Design review of the part shown in the three views and the two pictorial views. Dimensions are in mm from the part's minimum x, y and z. Round coordinates to 2 decimals unless told otherwise and drop trailing zeros. Loops run counter-clockwise (first coordinate to the right, second up) from the corner with the lowest first, then second, coordinate; pieces in that order, holes last.
1) Insertion check: pin 1 (8 mm diameter, centred on x = 7, y = 21, fed in from -Z); pin 2 (0.5 mm diameter, centred on y = 7, z = 0.5, fed in from -X). Each pin has a flat end and moves straight along its axis. Give the tip position at first contact, or say it passes through.
2) Take a section at A-A (z = 0.3). State the section outline as (x, y) points, then the cut area to 3 significant figures.
3) Take a section at B-B (y = 12.75). State the section outline as (x, z) points, then the cut area to 3 significant figures.
4) Wall thickness on L1, parallel to X at y = 2.75, z = 0.6; L2, parallel to Y at x = 2.5, z = 0.25: over which ranges is each line inside the solid? List them lowest first.
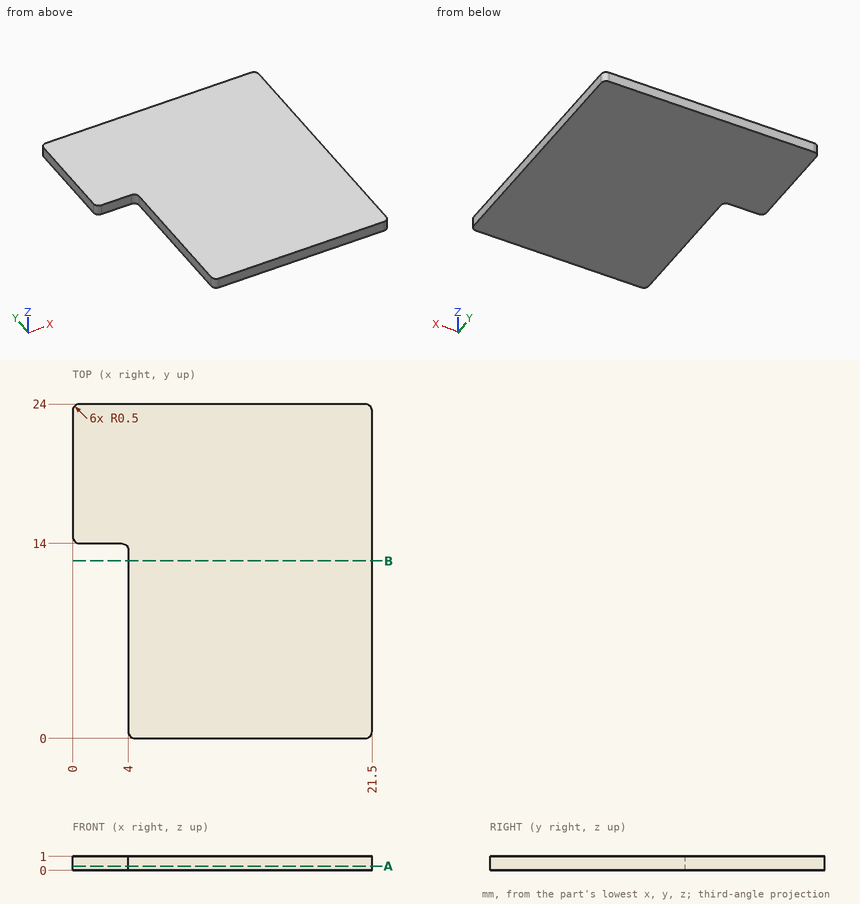
Response:
1. pin 1: stops at z = 0
1. pin 2: stops at x = 4
2. outline: (0, 14.5) arc R0.5 ccw to (0.5, 14) - (3.5, 14) arc R0.5 cw to (4, 13.5) - (4, 0.5) arc R0.5 ccw to (4.5, 0) - (21, 0) arc R0.5 ccw to (21.5, 0.5) - (21.5, 23.5) arc R0.5 ccw to (21, 24) - (0.5, 24) arc R0.5 ccw to (0, 23.5) - close
2. area: 460 mm2
3. outline: (4, 0) - (21.5, 0) - (21.5, 1) - (4, 1) - close
3. area: 17.5 mm2
4. L1: x = 4 to 21.5
4. L2: y = 14 to 24
